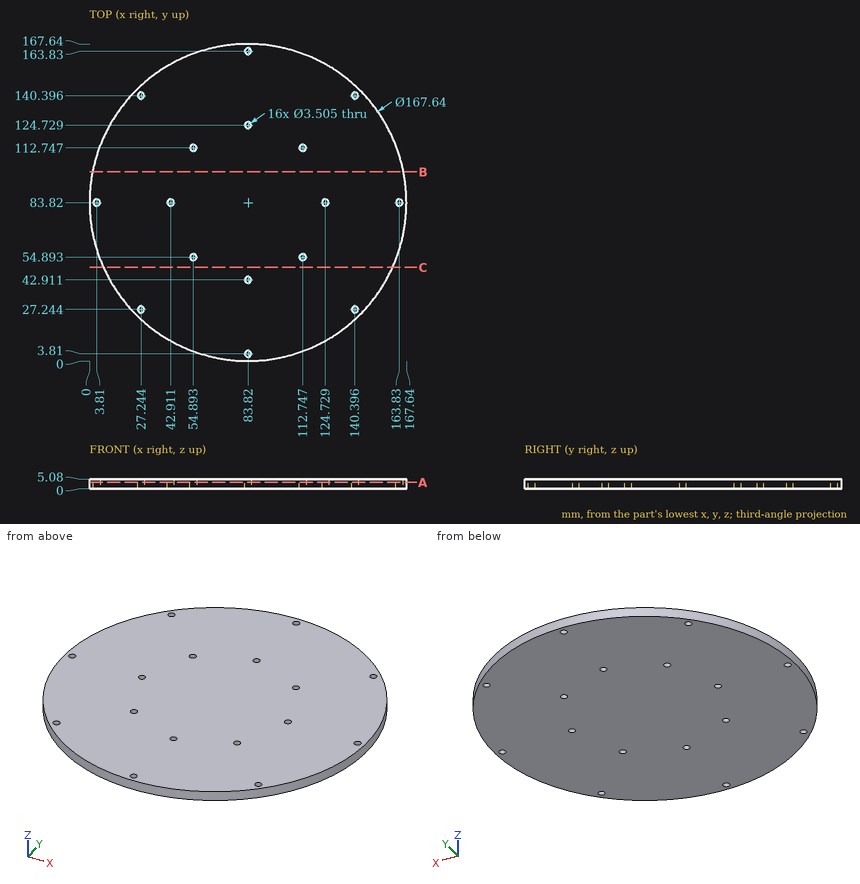
Geometry: see drawing. Coordinates: mm, zero at the bounding-box minimum. Coordinates: 2 decimals unless noted, no trailing zeros. Write each loop counter-clockwise with the first axis right and the second up, starting at its lowest first coordinate (ties: lowest second). Pieces come first, ordered by that corner, then holes.
1) Section C-C on y = 49.5. Output: boundary loops of the cut face in (x, z).
2) Material intervals for line 1 along Y through (x, z) = (83.82, 2.5); line 2 along Y through (x, z) = (26, 4.35) (1 decimal); line 3 along Y through (x, z) = (13.5, 0.5) (1 decimal), sorted ascending.
3) Section B-B on y = 100. Output: boundary loops of the cut face in (x, z).
4) Section A-A on z = 3.3. State how many separate pieces and enclosed holes the cut face has, and give its area (3 significant figures).
5) Pin query (flat end, axial travel): pin 1 Ø3 at (x, y) = (54.89, 112.75) entering from +Z; pin 2 Ø1.5 at (y, z) = (28, 3.5) entering from +X; pin 3 Ø1.5 at (y, z) = (102, 3) entering from +X. Return the tip coordinate at first contact, or that it passes through.
Check result:
1. outline: (7.35, 0) - (160.29, 0) - (160.29, 5.08) - (7.35, 5.08) - close
2. line 1: y = 0 to 2.06, 5.56 to 41.16, 44.66 to 122.98, 126.48 to 162.08, 165.58 to 167.64
2. line 2: y = 23.1 to 26, 28.5 to 139.2, 141.6 to 144.5
2. line 3: y = 38.2 to 129.4
3. outline: (1.58, 0) - (166.06, 0) - (166.06, 5.08) - (1.58, 5.08) - close
4. separate pieces: 1
4. enclosed holes: 16
4. area: 21,900 mm2
5. pin 1: passes through
5. pin 2: stops at x = 147.01
5. pin 3: stops at x = 165.81
